Part print with two shaded views. Sizes in mm from the minimum x, y, z corner. A direction names the side the tool comes from. Coordinates: 2 decimals unless noted, no trailing zeros. Loops run counter-clockwise (first coordinate to the right, second up) from the corner with the lowest first, then second, coordinate; pieces in that order, holes last. Notation, with made-up numbers: (5, -12.75) - (61, -12.75) arc R13 cw to (61, 12.25) - close; hole circle Ø7 at (37.5, 46). An arc over 180 degrees is marked (long way). Answer as CSV lines item,"result".
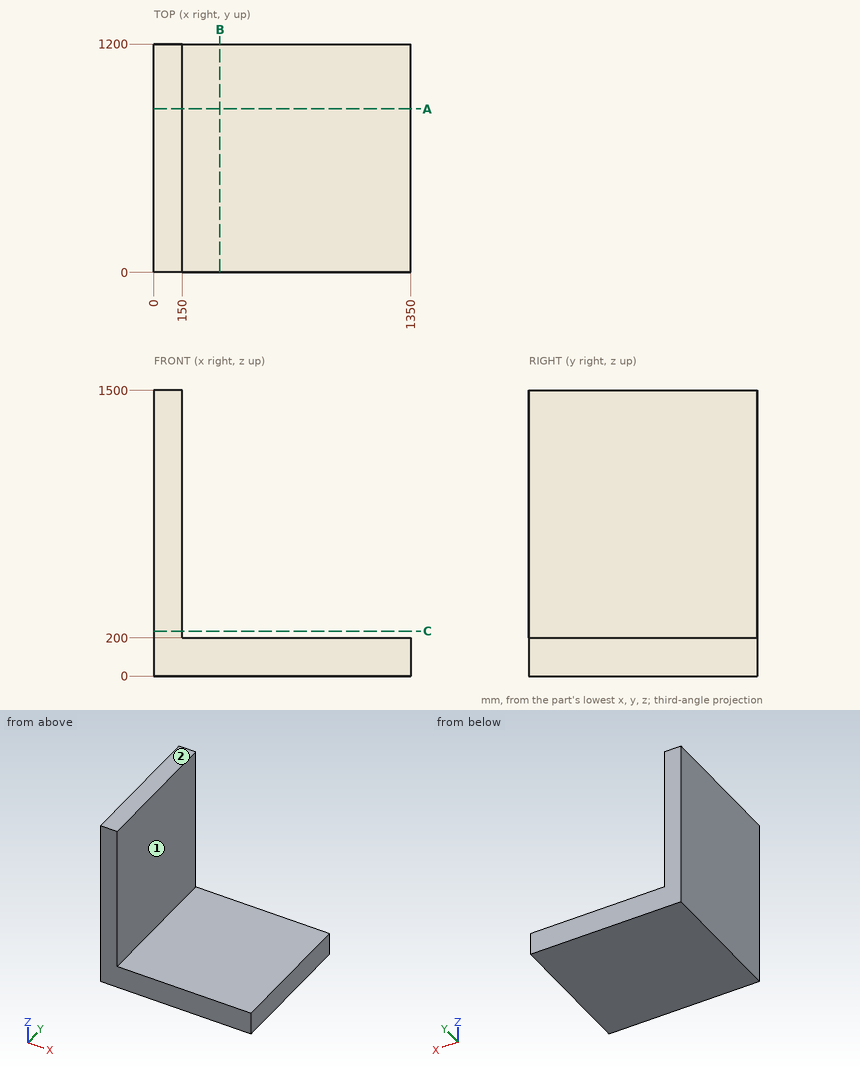
Q1. Flat gauge pins, fed straight in: pin 1 (8 mm diameter, centred on y = 250.5, z = 220, fed in from +X); pin 2 (2 mm diameter, centred on x = 651, y = 585.5, fed in from -Z). Where does each tip first touch, or does it go through?
Results:
pin 1,"stops at x = 150"
pin 2,"stops at z = 0"
Q2. Saw through at B-B (x = 347.5). Give the cut face in (y, z), then the cut area to 3 significant figures.
Results:
outline,"(0, 0) - (1200, 0) - (1200, 200) - (0, 200) - close"
area,"240,000 mm^2"
Q3. Which spindle directions (+Z, -Z, +X, -X, +Y, -Y) get a long thin tool onto all of the face, cutting with end or side? Do the marked faces 1 and 2. Say none if no direction does.
Results:
face 1,"+Z, +X, +Y, -Y"
face 2,"+Z, +X, -X, +Y, -Y"
Q4. Wall check: L1, parallel to Z at x = 1036, y = 644.5; L2, parallel to X at y = 130.5, z = 908.5. Give the ranges that are in metal, low to high.
Results:
L1,"z = 0 to 200"
L2,"x = 0 to 150"
Q5. Saw through at C-C (z = 236). Give the cut face in (x, y).
Results:
outline,"(0, 0) - (150, 0) - (150, 1200) - (0, 1200) - close"
Q6. Saw through at A-A (y = 859.5). Give the cut face in (x, z), then the cut area to 3 significant figures.
Results:
outline,"(0, 0) - (1350, 0) - (1350, 200) - (150, 200) - (150, 1500) - (0, 1500) - close"
area,"465,000 mm^2"
